Source: three-view drawing plus pictorial views. Frame: mm from the lowest corner of the part. Give positions to 0.01 mm unless a question says otherwise; leave off trailing zeros. Order: outer loops, then holes, each group sorted by start corner. A loop starts at its lowest first (then second) coordinate and runs counter-clockwise, first axis right, second up.
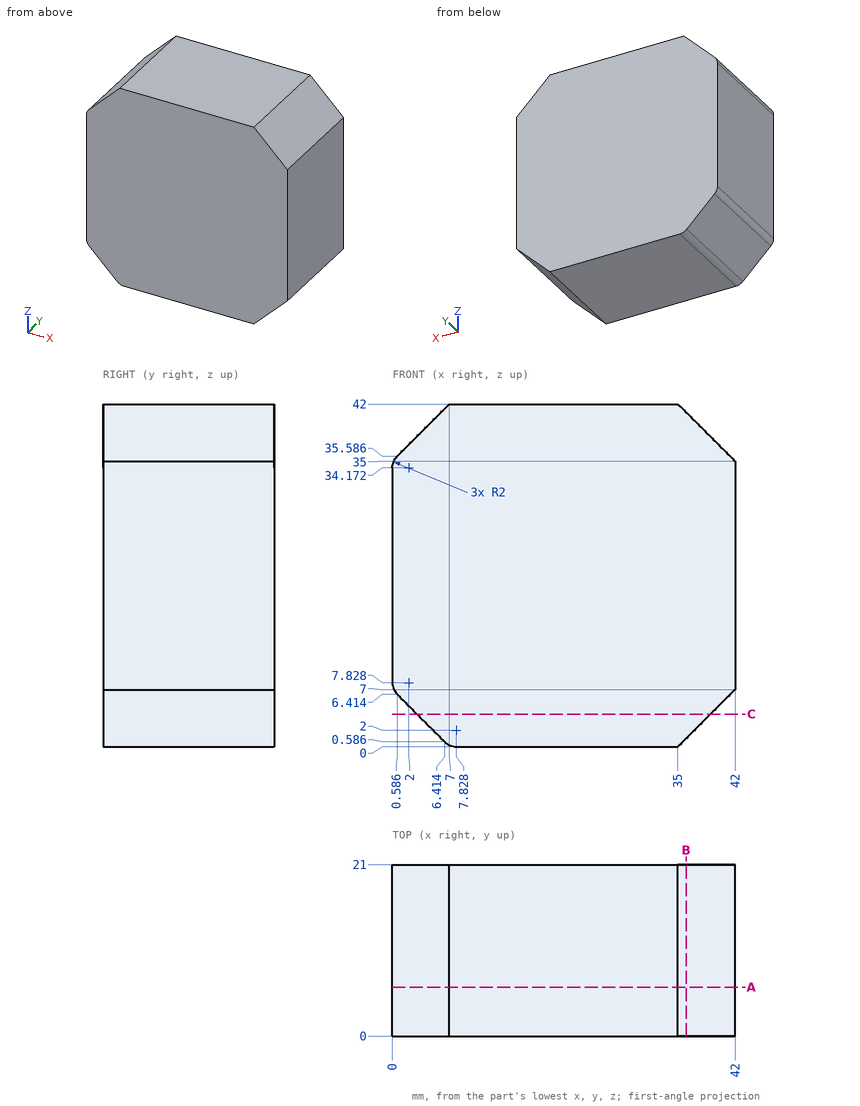
(1) Section B-B, the plane x = 36. Return loops of the section in (y, z), plus the area to 3 significant figures.
(2) Line query: line 1 along Z through (x, y) = (5, 19); line 2 along X through (y, z) = (15.25, 40); line 3 along X through (y, z) = (18, 7). Output: solid intervals per line, ascending.
(3) Section C-C, the plane z = 4. Return loops of the section in (x, y), plus the area to 3 significant figures.
(4) Pin query (flat end, axial travel): pin 1 Ø6 at (x, z) = (8, 30) entering from -Y; pin 2 Ø1.5 at (y, z) = (13.5, 6) entering from +X. Return the tip coordinate at first contact, or that it passes through.
(5) Section A-A, the plane y = 6. Return loops of the section in (x, z) (1 decimal), plus the area to 3 significant figures.
Checks:
1. outline: (0, 1) - (21, 1) - (21, 41) - (0, 41) - close
1. area: 840 mm2
2. line 1: z = 2 to 40
2. line 2: x = 5 to 37
2. line 3: x = 0.18 to 42
3. outline: (3, 0) - (39, 0) - (39, 21) - (3, 21) - close
3. area: 756 mm2
4. pin 1: stops at y = 0
4. pin 2: stops at x = 41.75
5. outline: (0, 7.8) arc R2 ccw to (0.6, 6.4) - (6.4, 0.6) arc R2 ccw to (7.8, 0) - (35, 0) - (42, 7) - (42, 35) - (35, 42) - (7, 42) - (0.6, 35.6) arc R2 ccw to (0, 34.2) - close
5. area: 1,670 mm2
